Autodesk Inventor part; units mm, degrees
ref_plane "YZ Plane" through (0, 0, 0) normal (1, 0, 0) x (0, 1, 0)
ref_plane "XZ Plane" through (0, 0, 0) normal (0, 1, 0) x (-1, 0, 0)
ref_plane "XY Plane" through (0, 0, 0) normal (0, 0, 1) x (1, 0, 0)
sketch "Esboço1" plane through (0, 0, 0) normal (0, 0, 1) x (1, 0, 0)
  line L0 (0, 306.9957) -> (70, 306.9957)
  line L1 (140, 226.9957) -> (140, -33.0043)
  line L2 (140, -33.0043) -> (0, -33.0043)
  line L3 (0, -33.0043) -> (0, 306.9957)
  line L4 (70, 306.9957) -> (140, 226.9957)
  dimension "d0" = 140
  dimension "d1" = 340
  dimension "d2" = 70
  dimension "d3" = 260
extrude "Extrusão1" add sketch "Esboço1" along normal blind 15.88
sketch "Esboço3" plane through (0, 0, 0) normal (0, 0, -1) x (-1, 0, 0)
  line L0 (0, 21.9457) -> (-140, 21.9457)
  line L1 (0, 21.9457) -> (0, 37.9257)
  line L2 (-140, 37.9257) -> (0, 37.9257)
  line L3 (-140, 21.9457) -> (-140, 37.9257)
  line L4 (-140, -33.0043) -> (-140, 226.9957) construction
  line L5 (-140, 29.9357) -> (0, 29.9357) construction
  point P0 (0, 0)
  dimension "d11" = 15.98
extrude "Extrusão3" cut sketch "Esboço3" against normal blind 3
sketch "Esboço4" plane through (0, 0, 0) normal (0, 0, -1) x (-1, 0, 0)
  circle A0 centre (-82, 12.9957) radius 2.1
  circle A1 centre (-82, 12.9957) radius 2.1
  circle A2 centre (-58, 12.9957) radius 2.1
  circle A3 centre (-58, -27.0043) radius 2.1
  circle A4 centre (-82, -27.0043) radius 2.1
  point P0 (0, 0)
hole "Furo1" at (82, 12.9957, 0) at (82, 12.9957, 0) at (58, 12.9957, 0) at (58, -27.0043, 0) at (82, -27.0043, 0) direction (0, 0, 1) diameter 5.5 end through all counterbore diameter 8 counterbore depth 6
properties part number "LATERAL_BLOCOS_BASE"
CAD build for the part. Positions are in the model's coordinates, mm. A direction names the side the tool comes from. Round coordinates to 2 decimals unless told otherwise and drop trailing zeros. Write each loop counter-clockwise with the first axis right and the second up, starting at its lowest first coordinate (ties: lowest second). Pieces come first, ordered by that corner, then holes. Notation, with made-up numbers: M 36,67 L 51,67 A29 cw 51,94 Z; hole C 84.25,37.5 d8. An arc over 180 degrees is marked long. Use a Markdown table: item, result. Add a question column.
1. 3-axis set-ups, long thin cutter, end or side, ignore diameter. For faces 4 (the face through (71, 30, 3)), 5 (the face through (85.9, -27.9, 3)), 6 (the face through (71, -33.004, 8)): which of +Z, -Z, +X, -X, +Y, -Y reach the whole face in a straight line?
2. Slice it at A-A on z = 10. Give the cut face in (x, y).
3. Slice it at B-B on y = 268. Give the cut face in (x, z), then the cut area to 3 significant figures.
4. Pull direction Y, two halves, no side cores. Call faces 1 (the face through (61, 12, 6)), 2 (the face through (69, -5, 0)), 3 (the face through (35, 306.996, 8)): released by +Y, released by -Y, zero draft, split by the parting line, or undercut.
5. Drill centre lines: probe 1 along Y at (x, z) = (58, 4.5); probe 2 along Y at (x, z) = (58, 2.15); probe 3 along Y at (x, z) = (82, 1.8). Where is each one in solid material? Low to high.
6. Flat gauge pins, fed straight in: P1, Ø8, axis at x = 50, y = 30.5, coming from the -Z side; P2, Ø7, axis at x = 82, y = -27, coming from the -Z side; P3, Ø4.5, axis at x = 82, y = -27, coming from the +Z side; P4, Ø3.5, axis at x = 91.5, z = 2, coming from the +Y side. Where does each tip first touch, or does it go through?
Reply:
| question | item | result |
|---|---|---|
| 1 | face 4 | -Z, +X, -X |
| 1 | face 5 | -Z |
| 1 | face 6 | +Z, -Z, +X, -X, -Y |
| 2 | outline | M 0,-33 L 140,-33 L 140,227 L 70,307 L 0,307 Z; hole C 58,-27 d5.5; hole C 58,13 d5.5; hole C 82,-27 d5.5; hole C 82,13 d5.5 |
| 3 | outline | M 0,0 L 104.12,0 L 104.12,15.88 L 0,15.88 Z |
| 3 | area | 1,650 mm^2 |
| 4 | face 1 | undercut |
| 4 | face 2 | zero draft |
| 4 | face 3 | released by +Y |
| 5 | probe 1 | y = -33 to -31, -23 to 9, 17 to 307 |
| 5 | probe 2 | y = -33 to -31, -23 to 9, 17 to 21.95, 37.93 to 307 |
| 5 | probe 3 | y = -33 to -31, -23 to 9, 17 to 21.95, 37.93 to 293.28 |
| 6 | P1 | stops at z = 3 |
| 6 | P2 | stops at z = 6 |
| 6 | P3 | passes through |
| 6 | P4 | stops at y = 284.42 |
